Source: CAD feature listing. Evaluate the final solid. Frame: model axes, mm. Face numbers are marked on the shaded views. A direction names the side the tool comes from. Coordinates: 2 decimals unless noted, no trailing zeros. Order: outer loops, then holes, each group sorted by start corner. A loop starts at its lowest first (then second) coordinate and runs counter-clockwise, first axis right, second up.
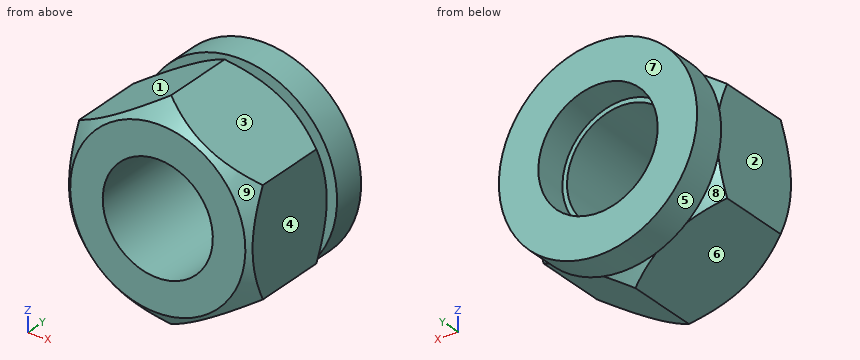
```python
from build123d import *

# Parameters (mm, degrees)
SZKIC1_R                    = 3
DODANIE_WYCI_GNI_CIE1_DEPTH = 3
SZKIC4_R                    = 5.4
SZKIC4_R_2                  = 3.25
DODANIE_WYCI_GNI_CIE2_DEPTH = 1.8


with BuildPart() as part:
    # Szkic1 → Dodanie-wyciągnięcie1 (new, symmetric)
    with BuildSketch(Plane(origin=(0, 0, 0), x_dir=(1, 0, 0), z_dir=(0, 1, 0))):
        Polygon((5, -2.886751346), (5, 2.886751346), (0, 5.773502692), (-5, 2.886751346), (-5, -2.886751346), (0, -5.773502692), align=None)
        with Locations(Location((0, 0, 0), (0, 0, 270))):
            Circle(SZKIC1_R, mode=Mode.SUBTRACT)
    extrude(amount=DODANIE_WYCI_GNI_CIE1_DEPTH, both=True)

    # Szkic3 → Wycięcie-obrót9 (revolve, cut)
    with BuildSketch(Plane(origin=(0, 0, 0), x_dir=(0, 0, -1), z_dir=(1, 0, 0)), mode=Mode.PRIVATE) as wyci_cie_obr_t9_sk:
        Polygon((5.773502692, 3), (5.773502692, 2), (4.773502692, 3), align=None)
        Polygon((4.773502692, -3), (5.773502692, -3), (5.773502692, -2), align=None)
    revolve(wyci_cie_obr_t9_sk.sketch.rotate(Axis((0, 0, 0), (0, 1, 0)), 180), axis=Axis((0, 0, 0), (0, 1, 0)), mode=Mode.SUBTRACT)

    # Szkic4 → Dodanie-wyciągnięcie2 (add)
    with BuildSketch(Plane(origin=(0, 3, 0), x_dir=(1, 0, 0), z_dir=(0, 1, 0))):
        with Locations(Location((0, 0, 0), (0, 0, 270))):
            Circle(SZKIC4_R)
        with Locations(Location((0, 0, 0), (0, 0, 270))):
            Circle(SZKIC4_R_2, mode=Mode.SUBTRACT)
    extrude(amount=DODANIE_WYCI_GNI_CIE2_DEPTH)


solid = part.part
```
1. Section query B-B, the plane y = -1.5. Output: boundary loops of the cut face in (x, z), plus the area to 3 significant figures.
2. Draft query along Y for the marked faces 6, 7, 8 and 9. Return one class per face: +Y half, -Y half, draft (parallel to the pull), parting line (faces both ways), or undercut.
3. Section query A-A, the plane z = 0. Output: boundary loops of the cut face in (x, y).
4. Access query for the marked faces 1, 2, 3, 4 and 5. Directions: +Z, -Z, +X, -X, +Y, -Y. A direction counts if a zero-diameter tool reaches every point of the face in a straight line with its end or side. Return the directions, or none.
5. Material intervals for line 1 along X through (y, z) = (1.1, 0); line 2 along Y through (x, z) = (-4, -3); line 3 along X through (y, z) = (4.15, 0), sorted ascending.
6. Contact query for flat-ended pins moving along their axis: P1, Ø1.7, axis at y = 0, z = -0.5, coming from the -X side; P2, Ø4, axis at x = 2.5, y = -2, coming from the +Z side; P3, Ø1.5, axis at x = -2, y = 1.5, coming from the +Z side. Output: stop coordinate, or through.
Answer key:
1. outline: (-5, -2.89) - (0, -5.77) - (5, -2.89) - (5, 2.89) - (0, 5.77) - (-5, 2.89) - close; hole circle Ø6 at (0, 0)
1. area: 58.3 mm2
2. face 6: draft
2. face 7: +Y half
2. face 8: undercut
2. face 9: -Y half
3. outline: (-5.4, 3) - (-4.77, 3) - (-5, 2.77) - (-5, -2.77) - (-4.77, -3) - (-3, -3) - (-3, 3) - (-3.25, 3) - (-3.25, 4.8) - (-5.4, 4.8) - close; (3, -3) - (4.77, -3) - (5, -2.77) - (5, 2.77) - (4.77, 3) - (5.4, 3) - (5.4, 4.8) - (3.25, 4.8) - (3.25, 3) - (3, 3) - close
4. face 1: +Z, -X, -Y
4. face 2: +Z, -Z, -X, -Y
4. face 3: +Z, +X, -Y
4. face 4: +Z, -Z, +X, -Y
4. face 5: +Y
5. line 1: x = -5 to -3, 3 to 5
5. line 2: y = -2.77 to 2.77, 3 to 4.8
5. line 3: x = -5.4 to -3.25, 3.25 to 5.4
6. P1: stops at x = -5
6. P2: stops at z = 5.48
6. P3: stops at z = 5.05
